Check sheet for the modelled part. Datum: model origin and axes. Units: mm. A direction names the side the tool comes from. Round coordinates to 2 decimals unless told otherwise and drop trailing zeros. Order: outer loops, then holes, each group sorted by start corner. A loop starts at its lowest first (then second) coordinate and runs counter-clockwise, first axis right, second up. Notation, with made-up numbers: (-7, -1) -> (-1, -1) arc R7 cw to (-1, 3) -> close; hole circle Ø4 at (3, 57.25). An arc over 180 degrees is marked (long way). Answer as CSV lines item,"result". Start each with the question number.
from build123d import *

# Parameters (mm, degrees)
SKETCH_1_W          = 87
SKETCH_1_H          = 71
EXTRUDE_1_DEPTH     = 2
SKETCH_2_W          = 91
SKETCH_2_H          = 75
SKETCH_2_W_2        = 87
SKETCH_2_H_2        = 71
EXTRUDE_2_DEPTH     = 17
SKETCH_3_R          = 4.25
CUT_EXTRUDE_2_DEPTH = 17
SKETCH_4_W          = 91
SKETCH_4_H          = 75
SKETCH_4_W_2        = 89
SKETCH_4_H_2        = 73
EXTRUDE_3_DEPTH     = 17
SKETCH_6_W          = 16
SKETCH_6_H          = 9
CUT_EXTRUDE_3_DEPTH = 17
SKETCH_7_W          = 21
SKETCH_7_H          = 7
CUT_EXTRUDE_4_DEPTH = 17
EXTRUDE_4_DEPTH     = 3
EXTRUDE_5_DEPTH     = 3


with BuildPart() as part:
    # 草图1 → 凸台-拉伸1 (new body)
    with BuildSketch(Plane(origin=(0, 0, 0), x_dir=(1, 0, 0), z_dir=(0, 1, 0))):
        Rectangle(SKETCH_1_W, SKETCH_1_H)
    extrude(amount=EXTRUDE_1_DEPTH)

    # 草图2 → 凸台-拉伸2 (add)
    with BuildSketch(Plane(origin=(0, 0, 0), x_dir=(1, 0, 0), z_dir=(0, 1, 0))):
        Rectangle(SKETCH_2_W, SKETCH_2_H)
        Rectangle(SKETCH_2_W_2, SKETCH_2_H_2, mode=Mode.SUBTRACT)
    extrude(amount=EXTRUDE_2_DEPTH)

    # 草图3 → 切除-拉伸2 (cut)
    with BuildSketch(Plane(origin=(45.5, 0, 0), x_dir=(0, 0, -1), z_dir=(1, 0, 0))):
        with Locations((-30.5, 9)):
            Circle(SKETCH_3_R)
    extrude(amount=-CUT_EXTRUDE_2_DEPTH, mode=Mode.SUBTRACT)

    # 草图4 → 凸台-拉伸3 (add)
    with BuildSketch(Plane(origin=(0, 17, 0), x_dir=(1, 0, 0), z_dir=(0, 1, 0))):
        Rectangle(SKETCH_4_W, SKETCH_4_H)
        Rectangle(SKETCH_4_W_2, SKETCH_4_H_2, mode=Mode.SUBTRACT)
    extrude(amount=EXTRUDE_3_DEPTH)

    # 草图6 → 切除-拉伸3 (cut)
    with BuildSketch(Plane.ZY.offset(45.5)):
        with Locations((28.5, 21.5)):
            Rectangle(SKETCH_6_W, SKETCH_6_H)
    extrude(amount=-CUT_EXTRUDE_3_DEPTH, mode=Mode.SUBTRACT)

    # 草图7 → 切除-拉伸4 (cut)
    with BuildSketch(Plane.XY.offset(37.5)):
        with Locations((-16, 20.5)):
            Rectangle(SKETCH_7_W, SKETCH_7_H)
    extrude(amount=-CUT_EXTRUDE_4_DEPTH, mode=Mode.SUBTRACT)

    # 草图8 → 凸台-拉伸4 (add)
    with BuildSketch(Plane.ZY.offset(45.5)):
        Polygon((-37.5, 17), (-37.5, 23), (-29.5, 23), align=None)
        Polygon((-20.5, 23), (-28.5, 17), (-28.5, 23), align=None)
        Polygon((-11.5, 23), (-19.5, 17), (-19.5, 23), align=None)
        Polygon((-2.5, 23), (-10.5, 17), (-10.5, 23), align=None)
        Polygon((6.5, 23), (-1.5, 17), (-1.5, 23), align=None)
        Polygon((15.5, 23), (7.5, 17), (7.5, 23), align=None)
    extrude(amount=EXTRUDE_4_DEPTH)

    # 草图9 → 凸台-拉伸5 (add)
    with BuildSketch(Plane(origin=(45.5, 0, 0), x_dir=(0, 0, -1), z_dir=(1, 0, 0))):
        Polygon((37.5, 23), (29.5, 23), (29.5, 17), align=None)
        Polygon((20.5, 17), (28.5, 23), (20.5, 23), align=None)
        Polygon((11.5, 17), (19.5, 23), (11.5, 23), align=None)
        Polygon((2.5, 17), (10.5, 23), (2.5, 23), align=None)
        Polygon((-6.5, 17), (1.5, 23), (-6.5, 23), align=None)
        Polygon((-15.5, 17), (-7.5, 23), (-15.5, 23), align=None)
    extrude(amount=EXTRUDE_5_DEPTH)


solid = part.part
1) Section check D-D on z = 17. Record the cut outline in (x, y), then the cut area to 3 significant figures.
2) Access from +Z, -Z, +X, -X, +Y, -Y to the whole of each face (thin tool, end or side, straight path). Record for faces 1 (the face through (46.979, 19.958, -6.444)), 2 (the face through (-47, 20, -19.5)), 3 (the face through (-1, 25, -36.5)).
3) Section check A-A on z = 30.5. Record the cut outline in (x, y).
4) Material ranges on line 1 along X through (y, z) = (26, -21.5); line 2 along X through (y, z) = (14, 14); line 3 along Z through (x, y) = (5, 22.5), recorded low to high.
5) Mould release check, pull along X, two halves, no side actions. Record for faces 4 (the face through (46.979, 19.958, 11.556)), 5 (the face through (-48.5, 21, 10)), 6 (the face through (-1, 9, 35.5)), 7 (the face through (-1, 9, -35.5)): released by +X, released by -X, zero draft, split by the parting line, or undercut.
6) Section check C-C on y = 9. Record the cut outline in (x, z), then the cut area to 3 significant figures.
7) Depth check by flat-ended pin: pin 1 Ø1.5 at (x, y) = (47, 20) entering from +Z; pin 2 Ø10 at (x, z) = (-21.5, -3) entering from -Y; pin 3 Ø2.5 at (x, z) = (47, -25) entering from +Y; pin 4 Ø0.8 at (y, z) = (20.5, 37) entering from -X. Enter the tip coordinate at first touch or a pass-through.
8) Section check B-B on x = -18.5. Record the cut outline in (y, z).
Solutions:
1,outline,"(-45.5, 0) -> (45.5, 0) -> (45.5, 34) -> (44.5, 34) -> (44.5, 17) -> (43.5, 17) -> (43.5, 2) -> (-43.5, 2) -> (-43.5, 17) -> (-44.5, 17) -> (-44.5, 34) -> (-45.5, 34) -> close"
1,area,"276 mm^2"
2,face 1,"+X, -Y"
2,face 2,"-X, +Y, -Y"
2,face 3,"+Y"
3,outline,"(-45.5, 0) -> (45.5, 0) -> (45.5, 4.75) -> (43.5, 4.75) -> (43.5, 2) -> (-43.5, 2) -> (-43.5, 17) -> (-45.5, 17) -> close; (-45.5, 26) -> (-44.5, 26) -> (-44.5, 34) -> (-45.5, 34) -> close; (43.5, 13.25) -> (45.5, 13.25) -> (45.5, 34) -> (44.5, 34) -> (44.5, 17) -> (43.5, 17) -> close"
4,line 1,"x = -45.5 to -44.5, 44.5 to 45.5"
4,line 2,"x = -45.5 to -43.5, 43.5 to 45.5"
4,line 3,"z = -37.5 to -36.5, 36.5 to 37.5"
5,face 4,"zero draft"
5,face 5,"released by -X"
5,face 6,"undercut"
5,face 7,"undercut"
6,outline,"(-45.5, -37.5) -> (45.5, -37.5) -> (45.5, 26.25) -> (43.5, 26.25) -> (43.5, -35.5) -> (-43.5, -35.5) -> (-43.5, 35.5) -> (43.5, 35.5) -> (43.5, 34.75) -> (45.5, 34.75) -> (45.5, 37.5) -> (-45.5, 37.5) -> close"
6,area,"631 mm^2"
7,pin 1,"stops at z = 15.5"
7,pin 2,"stops at y = 0"
7,pin 3,"stops at y = 23"
7,pin 4,"stops at x = -45.5"
8,outline,"(0, -37.5) -> (34, -37.5) -> (34, -36.5) -> (17, -36.5) -> (17, -35.5) -> (2, -35.5) -> (2, 35.5) -> (17, 35.5) -> (17, 37.5) -> (0, 37.5) -> close; (24, 36.5) -> (34, 36.5) -> (34, 37.5) -> (24, 37.5) -> close"
